from build123d import *

# Parameters (mm, degrees)
SKETCH1_R           = 20
SKETCH1_R_2         = 5
BOSS_EXTRUDE2_DEPTH = 10


with BuildPart() as part:
    # Sketch1 → Boss-Extrude2 (new body)
    with BuildSketch(Plane(origin=(0, 0, 0), x_dir=(1, 0, 0), z_dir=(0, 1, 0))):
        with BuildLine():
            Line((-55, -7.5), (-43.229041164, -7.5))
            ThreePointArc((-43.229041164, -7.5), (-40.224415102, -8.503473731), (-38.425814368, -11.111111111))
            ThreePointArc((-38.425814368, -11.111111111), (0, -40), (38.425814368, -11.111111111))
            ThreePointArc((38.425814368, -11.111111111), (40.224415102, -8.503473731), (43.229041164, -7.5))
            Line((43.229041164, -7.5), (55, -7.5))
            ThreePointArc((55, -7.5), (62.5, 0), (55, 7.5))
            Line((55, 7.5), (43.229041164, 7.5))
            ThreePointArc((43.229041164, 7.5), (40.224415102, 8.503473731), (38.425814368, 11.111111111))
            ThreePointArc((38.425814368, 11.111111111), (0, 40), (-38.425814368, 11.111111111))
            ThreePointArc((-38.425814368, 11.111111111), (-40.224415102, 8.503473731), (-43.229041164, 7.5))
            Line((-43.229041164, 7.5), (-55, 7.5))
            ThreePointArc((-55, 7.5), (-62.5, 0), (-55, -7.5))
        make_face()
        with Locations(Location((0, 0, 0), (0, 0, 270))):
            Circle(SKETCH1_R, mode=Mode.SUBTRACT)
        with Locations(Location((55, 0, 0), (0, 0, 270))):
            Circle(SKETCH1_R_2, mode=Mode.SUBTRACT)
        with Locations(Location((-55, 0, 0), (0, 0, 90))):
            Circle(SKETCH1_R_2, mode=Mode.SUBTRACT)
        with Locations(Location((10.383511712, 28.145740078, 0), (0, 0, 270))):
            Circle(SKETCH1_R_2, mode=Mode.SUBTRACT)
        with Locations(Location((-10.383511712, 28.145740078, 0), (0, 0, 90))):
            Circle(SKETCH1_R_2, mode=Mode.SUBTRACT)
        with Locations(Location((10.383511712, -28.145740078, 0), (0, 0, 90))):
            Circle(SKETCH1_R_2, mode=Mode.SUBTRACT)
        with Locations(Location((-10.383511712, -28.145740078, 0), (0, 0, 270))):
            Circle(SKETCH1_R_2, mode=Mode.SUBTRACT)
    extrude(amount=BOSS_EXTRUDE2_DEPTH)


solid = part.part
Verification items for the finished model (mm, model axes). A direction names the side the tool comes from. Give positions to 0.01 mm unless a question says otherwise; leave off trailing zeros. Write each loop counter-clockwise with the first axis right and the second up, starting at its lowest first coordinate (ties: lowest second). Pieces come first, ordered by that corner, then holes. Notation, with made-up numbers: (18.25, 2) -> (33.25, 2) arc R21 ccw to (33.25, 37) -> close; hole circle Ø11 at (35.25, 30.5). An arc over 180 degrees is marked (long way). Use CSV: the item, a comma, the result in double quotes.
(1) Go/stop test with flat-tipped pins: pin 1 (11.5 mm diameter, centred on x = -55, z = 0, fed in from -Y); pin 2 (1.5 mm diameter, centred on y = 4, z = 29.5, fed in from +X); pin 3 (2 mm diameter, centred on y = 8.5, z = -5, fed in from -X); pin 4 (3 mm diameter, centred on x = -46.5, y = 6, fed in from -Z). Record where each tip stops, or that it passes through.
Derived:
pin 1,"stops at y = 0"
pin 2,"stops at x = 27.81"
pin 3,"stops at x = -61.34"
pin 4,"stops at z = -7.5"
(2) Set-up check for faces 4 (the cylindrical face through (-19.524, 4.93, -4.336)), 5 (the flat face through (49, 5, -7.5)): record each of +Z, -Z, +X, -X, +Y, -Y from which the full face is reachable in a straight line by a thin tool's end or side.
Derived:
face 4,"+Y, -Y"
face 5,"-Z, +X, +Y, -Y"
(3) Release check for a two-part mould opening along Z. For faces 1 (the flat face through (49, 5, 7.5)), 2 (the cylindrical face through (59.957, 4.93, -0.651)), 3 (the flat face through (-10, 0, 18)) record: +Z half, -Z half, draft (parallel to the pull), parting line (faces both ways), or undercut.
Derived:
face 1,"+Z half"
face 2,"undercut"
face 3,"draft"
(4) Sectioned sample at B-B (y = 4). Record the cut outline in (x, z), plus the area to 3 significant figures.
Derived:
outline,"(-55, -7.5) -> (-43.23, -7.5) arc R5 cw to (-38.43, -11.11) arc R40 ccw to (38.43, -11.11) arc R5 cw to (43.23, -7.5) -> (55, -7.5) arc R7.5 ccw to (55, 7.5) -> (43.23, 7.5) arc R5 cw to (38.43, 11.11) arc R40 ccw to (-38.43, 11.11) arc R5 cw to (-43.23, 7.5) -> (-55, 7.5) arc R7.5 ccw to start; hole circle Ø10 at (-55, 0); hole circle Ø40 at (0, 0); hole circle Ø10 at (-10.38, -28.15); hole circle Ø10 at (-10.38, 28.15); hole circle Ø10 at (10.38, -28.15); hole circle Ø10 at (10.38, 28.15); hole circle Ø10 at (55, 0)"
area,"3,940 mm^2"
(5) Material ranges on L1, parallel to X at y = 7, z = 0; L2, parallel to X at y = 1.5, z = -4; L3, parallel to Z at x = -55, y = 6.75, recorded low to high.
Derived:
L1,"x = -62.5 to -60, -50 to -20, 20 to 50, 60 to 62.5"
L2,"x = -61.34 to -58, -52 to -19.6, 19.6 to 52, 58 to 61.34"
L3,"z = -7.5 to -5, 5 to 7.5"
(6) Sectioned sample at C-C (x = 3.5). Record the cut outline in (y, z), plus the area to 3 significant figures.
Derived:
outline,"(0, -39.85) -> (10, -39.85) -> (10, -19.69) -> (0, -19.69) -> close; (0, 19.69) -> (10, 19.69) -> (10, 39.85) -> (0, 39.85) -> close"
area,"403 mm^2"
(7) Sectioned sample at D-D (z = -29.5). Record the cut outline in (x, y), plus the area to 3 significant figures.
Derived:
outline,"(-27.01, 0) -> (-15.2, 0) -> (-15.2, 10) -> (-27.01, 10) -> close; (-5.57, 0) -> (5.57, 0) -> (5.57, 10) -> (-5.57, 10) -> close; (15.2, 0) -> (27.01, 0) -> (27.01, 10) -> (15.2, 10) -> close"
area,"348 mm^2"
(8) Sectioned sample at A-A (z = 0). Record the cut outline in (x, y).
Derived:
outline,"(-62.5, 0) -> (-60, 0) -> (-60, 10) -> (-62.5, 10) -> close; (-50, 0) -> (-20, 0) -> (-20, 10) -> (-50, 10) -> close; (20, 0) -> (50, 0) -> (50, 10) -> (20, 10) -> close; (60, 0) -> (62.5, 0) -> (62.5, 10) -> (60, 10) -> close"
